Read the model definition and answer for the solid it produces. Units are mm, in the model's axes. Face numbers are marked on the shaded views. A direction names the side the tool comes from. Coordinates: 2 decimals unless noted, no trailing zeros. Write each loop counter-clockwise with the first axis right and the second up, starting at its lowest first coordinate (ties: lowest second). Pieces come first, ordered by that corner, then holes. Notation, with made-up numbers: (44.25, 67) - (73.25, 67) arc R26 cw to (73.25, 91) - close; hole circle Ø9 at (-37, 39). An arc over 180 degrees is marked (long way). Use a Markdown table: item, result.
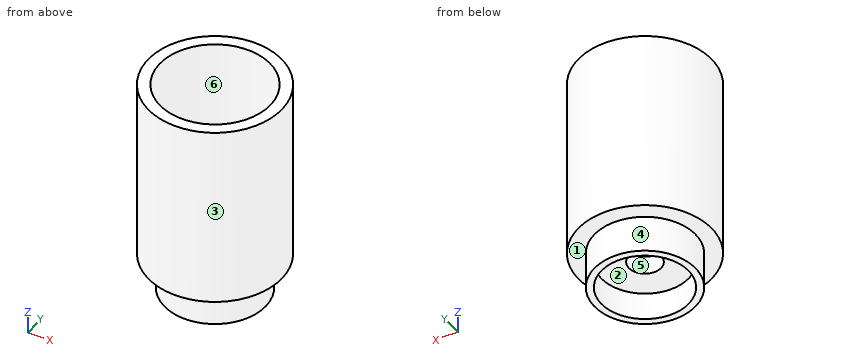
from build123d import *

# Parameters (mm, degrees)
SKETCH_1_R          = 14.5
EXTRUDE_1_DEPTH     = 40
SKETCH_2_R          = 12
CUT_EXTRUDE_1_DEPTH = 32
SKETCH_3_R          = 11
EXTRUDE_2_DEPTH     = 8
SKETCH_4_R          = 9.5
CUT_EXTRUDE_2_DEPTH = 6
CUT_EXTRUDE_START   = -6
SKETCH_5_R          = 9.5
CUT_EXTRUDE_3_DEPTH = 6
SKETCH_6_R          = 3.5
CUT_EXTRUDE_4_DEPTH = 6


with BuildPart() as part:
    # 스케치1 → 돌출1 (new body)
    with BuildSketch(Plane.XY):
        Circle(SKETCH_1_R)
    extrude(amount=EXTRUDE_1_DEPTH)

    # 스케치2 → 컷-돌출1 (cut)
    with BuildSketch(Plane.XY.offset(40)):
        Circle(SKETCH_2_R)
    extrude(amount=-CUT_EXTRUDE_1_DEPTH, mode=Mode.SUBTRACT)

    # 스케치3 → 돌출2 (add)
    with BuildSketch(Plane(origin=(0, 0, 0), x_dir=(-1, 0, 0), z_dir=(0, 0, -1))):
        with Locations(Location((0, 0, 0), (0, 0, 180))):
            Circle(SKETCH_3_R)
    extrude(amount=EXTRUDE_2_DEPTH)

    # 스케치4 → 컷-돌출2 (cut)
    with BuildSketch(Plane.XY.offset(8)):
        Circle(SKETCH_4_R)
    extrude(amount=-CUT_EXTRUDE_2_DEPTH, mode=Mode.SUBTRACT)

    # 스케치5 → 컷-돌출3 (cut)
    with BuildSketch(Plane(origin=(0, 0, -8), x_dir=(-1, 0, 0), z_dir=(0, 0, -1)).offset(CUT_EXTRUDE_START)):
        with Locations(Location((0, 0, 0), (0, 0, 180))):
            Circle(SKETCH_5_R)
    extrude(amount=CUT_EXTRUDE_3_DEPTH, mode=Mode.SUBTRACT)

    # 스케치6 → 컷-돌출4 (cut)
    with BuildSketch(Plane(origin=(0, 0, -2), x_dir=(-1, 0, 0), z_dir=(0, 0, -1))):
        Circle(SKETCH_6_R)
    extrude(amount=-CUT_EXTRUDE_4_DEPTH, mode=Mode.SUBTRACT)


solid = part.part
(1) For the marked faces 4, 5 and 6, determine the directions among +Z, -Z, +X, -X, +Y, -Y from which every point of the face is accessible in a straight line to the end or side of a thin tool.
Report:
| item | result |
|---|---|
| face 4 | -Z |
| face 5 | +Z, -Z |
| face 6 | +Z |
(2) A cutting plane is placed at A-A, the plane x = 0. Write down the section's boundary in (y, z).
Report:
| item | result |
|---|---|
| outline | (-14.5, 0) - (-11, 0) - (-11, -8) - (-9.5, -8) - (-9.5, -2) - (-3.5, -2) - (-3.5, 2) - (-9.5, 2) - (-9.5, 8) - (-12, 8) - (-12, 40) - (-14.5, 40) - close; (3.5, -2) - (9.5, -2) - (9.5, -8) - (11, -8) - (11, 0) - (14.5, 0) - (14.5, 40) - (12, 40) - (12, 8) - (9.5, 8) - (9.5, 2) - (3.5, 2) - close |
(3) Straight lines are drawn through the part: L1, parallel to Y at x = 0, z = 5.45; L2, parallel to Z at x = -11.25, y = -2; L3, parallel to Y at x = 0, z = 33. For each, find the intervals that lie inside material, in ascending order.
Report:
| item | result |
|---|---|
| L1 | y = -14.5 to -9.5, 9.5 to 14.5 |
| L2 | z = 0 to 8 |
| L3 | y = -14.5 to -12, 12 to 14.5 |
(4) The mould has two halves that part along X. Classify the marked faces 1, 2 and 3: pulls with the +X half, pulls with the -X half, needs draft (parallel to the pull), parting line crosses it, or undercut.
Report:
| item | result |
|---|---|
| face 1 | needs draft |
| face 2 | undercut |
| face 3 | parting line crosses it |
(5) Each of these flat-tipped pins is pushed along its axis until it touches: P1, Ø1, axis at y = -2, z = -2.5, coming from the -X side; P2, Ø5, axis at x = 4, z = 19.5, coming from the -Y side; P3, Ø17, axis at x = 0, y = 0, coming from the -Z side. Where does it stop, or does it pass through?
Report:
| item | result |
|---|---|
| P1 | stops at x = -10.9 |
| P2 | stops at y = -14.42 |
| P3 | stops at z = -2 |
(6) A cutting plane is placed at C-C, the plane z = 9.5. Write down the section's boundary in (x, y).
Report:
| item | result |
|---|---|
| outline | circle Ø29 at (0, 0); hole circle Ø24 at (0, 0) |
(7) A cutting plane is placed at D-D, the plane y = 7. Write down the section's boundary in (x, z), and give its area (3 significant figures).
Report:
| item | result |
|---|---|
| outline | (-12.7, 0) - (-8.49, 0) - (-8.49, -8) - (-6.42, -8) - (-6.42, -2) - (6.42, -2) - (6.42, -8) - (8.49, -8) - (8.49, 0) - (12.7, 0) - (12.7, 40) - (9.75, 40) - (9.75, 8) - (6.42, 8) - (6.42, 2) - (-6.42, 2) - (-6.42, 8) - (-9.75, 8) - (-9.75, 40) - (-12.7, 40) - close |
| area | 374 mm² |
